Model file for the job. Use its own axes, mm. Face numbers are marked on the shaded views. A direction names the side the tool comes from. Coordinates: 2 decimals unless noted, no trailing zeros. Loops run counter-clockwise (first coordinate to the right, second up) from the corner with the lowest first, then second, coordinate; pieces in that order, holes last. Notation, with made-up numbers: M 12,16 L 42,16 A12 cw 42,31 Z; hole C -4,11 d4. An arc over 180 degrees is marked long. One line per question, with ' | ' between items. Start each with the question number.
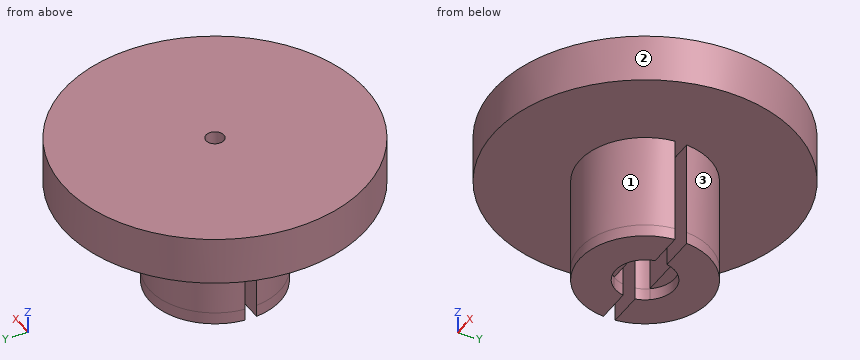
Autodesk Inventor part; units mm, degrees
ref_plane "YZ Plane" through (0, 0, 0) normal (1, 0, 0) x (0, 1, 0)
ref_plane "XZ Plane" through (0, 0, 0) normal (0, 1, 0) x (-1, 0, 0)
ref_plane "XY Plane" through (0, 0, 0) normal (0, 0, 1) x (1, 0, 0)
sketch "Sketch1" plane through (0, 0, 0) normal (0, 0, 1) x (1, 0, 0)
  circle A0 centre (0, 0) radius 2.5
  circle A1 centre (0, 0) radius 5.5
  dimension "d0" = 5
  dimension "d1" = 3
extrude "Extrusion1" add sketch "Sketch1" along normal blind 10
sketch "Sketch2" plane through (0, 0, 0) normal (0, 0, -1) x (-1, 0, 0)
  circle A0 centre (0, 0) radius 2.5 construction
  circle A1 centre (0, 0) radius 5.5 construction
  line L0 (-2, 1.5) -> (2, 1.5)
  circle A2 centre (0, 0) radius 2.5 construction
  line L1 (-2, -1.5) -> (2, -1.5)
  arc A3 (-2, 1.5) -> (-2, -1.5) centre (0, 0) ccw
  arc A4 (2, 1.5) -> (-2, 1.5) centre (0, 0) ccw
  arc A5 (2, -1.5) -> (2, 1.5) centre (0, 0) ccw
  arc A6 (-2, -1.5) -> (2, -1.5) centre (0, 0) ccw
  dimension "d4" = 3
extrude "Extrusion2" add sketch "Sketch2" against normal blind 10 contours A4 L0 | L1 A6
sketch "Sketch3" plane through (0, 0, 0) normal (1, 0, 0) x (0, 1, 0)
  line L0 (-1.5, 0) -> (1.5, 0) construction
  line L1 (1.5, 0) -> (-1.5, 0) construction
  line L2 (-5.5, 0) -> (5.5, 0) construction
  line L3 (1.5, 10) -> (-1.5, 10) construction
  line L4 (-1.5, 10) -> (1.5, 10) construction
  line L5 (5.5, 10) -> (-5.5, 10) construction
  line L6 (-0.5, 8) -> (0.5, 8)
  line L7 (0.5, 8) -> (0.5, 0)
  line L8 (0.5, 0) -> (-0.5, 0)
  line L9 (-0.5, 0) -> (-0.5, 8)
  point P0 (0, 0)
  point P1 (0, 10)
  point P2 (0, 8)
  dimension "d7" = 8
  dimension "d8" = 1
extrude "Extrusion3" cut sketch "Sketch3" along normal through all both and the other way through all
sketch "Sketch4" plane through (0, 0, 10) normal (0, 0, 1) x (1, 0, 0)
  arc A0 (2, -1.5) -> (2, 1.5) centre (0, 0) ccw
  line L0 (2, -1.5) -> (-2, -1.5)
  arc A1 (-2, 1.5) -> (-2, -1.5) centre (0, 0) ccw
  line L1 (-2, 1.5) -> (2, 1.5)
  circle A2 centre (0, 0) radius 5.5
extrude "Extrusion4" add sketch "Sketch4" against normal blind 2 contours L0 A1 L1 A0
sketch "Sketch5" plane through (0, 0, 10) normal (0, 0, 1) x (1, 0, 0)
  circle A0 centre (0, 0) radius 5.5
  circle A1 centre (0, 0) radius 12.7
  dimension "d13" = 25.4
extrude "Extrusion5" add sketch "Sketch5" against normal blind 2
sketch "Sketch6" plane through (0, 0, 0) normal (0, 0, -1) x (-1, 0, 0)
  line L0 (5.4772, -0.5) -> (2.4495, -0.5)
  arc A0 (2, -1.5) -> (2.4495, -0.5) centre (0, 0) ccw
  line L1 (2, -1.5) -> (-2, -1.5)
  arc A1 (-2.4495, -0.5) -> (-2, -1.5) centre (0, 0) ccw
  line L2 (-2.4495, -0.5) -> (-5.4772, -0.5)
  arc A2 (-5.4772, -0.5) -> (5.4772, -0.5) centre (0, 0) ccw
  line L3 (2.4495, 0.5) -> (5.4772, 0.5)
  arc A3 (5.4772, 0.5) -> (-5.4772, 0.5) centre (0, 0) ccw
  line L4 (-5.4772, 0.5) -> (-2.4495, 0.5)
  arc A4 (-2, 1.5) -> (-2.4495, 0.5) centre (0, 0) ccw
  line L5 (-2, 1.5) -> (2, 1.5)
  arc A5 (2.4495, 0.5) -> (2, 1.5) centre (0, 0) ccw
  circle A6 centre (0, 0) radius 2.5
extrude "Extrusion6" add sketch "Sketch6" along normal blind 1 contours A2 L2 A1 A6 A0 L0 | A6 L1 | A5 A6 A4 L4 A3 L3 | L5 A6
extrude "Extrusion7" cut sketch "Sketch6" along normal through all contours A0 L1 A1 A6 A4 L5 A5 | A6 L1 | L5 A6
sketch "Sketch7" plane through (0, 0, 10) normal (0, 0, 1) x (1, 0, 0)
  circle A0 centre (0, 0) radius 0.75
  dimension "d20" = 1.5
extrude "Extrusion8" cut sketch "Sketch7" against normal through all
sketch "Sketch8" plane through (0, 0, 10) normal (0, 0, 1) x (1, 0, 0)
  circle A0 centre (0, 0) radius 0.75
  circle A1 centre (0, 0) radius 12.7
extrude "Extrusion9" add sketch "Sketch8" along normal blind 2
properties part number "turntable"
(1) Band-saw the part on A-A on y = 0. Write the cut outline in (x, z).
(2) Pin check, flat tips, straight feed: P1, Ø3.5, axis at x = 3.5, z = 2.5, coming from the +Y side; P2, Ø3.5, axis at x = 3.5, z = 4.5, coming from the -Y side; P3, Ø2, axis at y = -3.5, z = 1, coming from the -X side. Stop position of each tip, or through.
(3) 3-axis set-ups, long thin cutter, end or side, ignore diameter. For the marked faces 1, 2 and 3: which of +Z, -Z, +X, -X, +Y, -Y reach the whole face in a straight line?
(4) Band-saw the part on D-D on y = 9.25. Write the cut outline in (x, z).
(5) Drill centre lines: line 1 (Y direction, x = 0, z = 9.95); line 2 (Y direction, x = 0, z = 5); line 3 (Z direction, x = 8, y = 2.5). Where is each one in solid material? Low to high. Write a range as [from, to].
Computed values:
1) outline: M -12.7,8 L -0.75,8 L -0.75,12 L -12.7,12 Z; M 0.75,8 L 12.7,8 L 12.7,12 L 0.75,12 Z
2) P1: y = 5.21 | P2: y = -5.21 | P3: x = -4.9
3) face 1: -Z, -Y | face 2: +Z, -Z | face 3: -Z, +Y
4) outline: M -8.7,8 L 8.7,8 L 8.7,12 L -8.7,12 Z
5) line 1: [-12.7, -0.75], [0.75, 12.7] | line 2: [-5.5, -1.5], [1.5, 5.5] | line 3: [8, 12]
